Autodesk Inventor part; units mm, degrees
ref_plane "YZ Plane" through (0, 0, 0) normal (1, 0, 0) x (0, 1, 0)
ref_plane "XZ Plane" through (0, 0, 0) normal (0, 1, 0) x (-1, 0, 0)
ref_plane "XY Plane" through (0, 0, 0) normal (0, 0, 1) x (1, 0, 0)
sketch "Sketch1" plane through (0, 0, 0) normal (0, 0, 1) x (1, 0, 0)
  line L0 (-23.7998, 0) -> (0, 0)
  line L1 (0, 0) -> (0, -127)
  line L2 (0, -127) -> (-23.7998, -127)
  line L3 (-23.7998, -127) -> (-23.7998, 0)
  circle A0 centre (-11.0998, -12.7) radius 1.7859
  circle A1 centre (-11.0998, -38.1) radius 1.7859
  circle A2 centre (-11.0998, -63.5) radius 1.7859
  circle A3 centre (-11.0998, -88.9) radius 1.7859
  circle A4 centre (-11.0998, -114.3) radius 1.7859
  line L4 (-11.0998, -12.7) -> (-11.0998, -38.1) construction
  line L5 (-11.0998, -38.1) -> (-11.0998, -63.5) construction
  line L6 (-11.0998, -63.5) -> (-11.0998, -88.9) construction
  line L7 (-11.0998, -88.9) -> (-11.0998, -114.3) construction
  dimension "d0" = 23.7998
  dimension "d1" = 127
  dimension "d2" = 3.5719
  dimension "d3" = 25.4
  dimension "d4" = 12.7
  dimension "d5" = 11.0998
extrude "Extrusion1" add sketch "Sketch1" along normal blind 1.5875
sketch "Sketch3" plane through (0, -127, 0) normal (1, 0, 0) x (0, 0, -1)
  line L0 (-25.3873, 127) -> (-1.5875, 127)
  line L1 (-1.5875, 127) -> (-1.5875, 0)
  line L2 (-1.5875, 0) -> (-25.3873, 0)
  line L3 (-25.3873, 0) -> (-25.3873, 127)
  circle A0 centre (-12.6873, 114.3) radius 1.7859
  circle A1 centre (-12.6873, 88.9) radius 1.7859
  circle A2 centre (-12.6873, 63.5) radius 1.7859
  circle A3 centre (-12.6873, 38.1) radius 1.7859
  circle A4 centre (-12.6873, 12.7) radius 1.7859
  line L4 (-12.6873, 114.3) -> (-12.6873, 88.9) construction
  line L5 (-12.6873, 88.9) -> (-12.6873, 63.5) construction
  line L6 (-12.6873, 63.5) -> (-12.6873, 38.1) construction
  line L7 (-12.6873, 38.1) -> (-12.6873, 12.7) construction
  dimension "d8" = 23.7998
  dimension "d9" = 127
  dimension "d10" = 3.5719
  dimension "d11" = 25.4
  dimension "d12" = 12.7
  dimension "d13" = 11.0998
extrude "Extrusion2" add sketch "Sketch3" along normal blind 1.5875
sketch "Sketch4" plane through (0, -127, 1.5875) normal (0, -1, 0) x (1, 0, 0)
  line L0 (0, 0) -> (1.5875, 0)
  line L1 (0, 23.7998) -> (1.5875, 23.7998)
  line L2 (1.5875, 0) -> (0, -1.5875)
  line L3 (0, -1.5875) -> (0, 0)
extrude "Extrusion3" add sketch "Sketch4" against normal blind 127
properties part number "Angle bracket"
Could you check a few things on this model? Use its own coordinates, in mm. A direction names the side the tool comes from. Coordinates: 2 decimals unless noted, no trailing zeros. Loops run counter-clockwise (first coordinate to the right, second up) from the corner with the lowest first, then second, coordinate; pieces in that order, holes last. Notation, with made-up numbers: M 53.5,-7 L 65.5,-7 A18 cw 65.5,13 Z; hole C 56.5,-22.5 d3. An arc over 180 degrees is marked long. Put each result on its own line as item: value. Start each with the question number.
(1) Suppose I cut it at C-C on z = 18.5. Please give me the cut outline in (x, y), then the cut area to 3 significant figures.
(2) Thinking about a two-plate mould opening in Y: for faces 1 (the face through (0.78, -116.07, 12.92)), 2 (the face through (1.588, -63, 16)), 3 (the face through (-6, -127, 1)), which applies, pulls with the +Y half, pulls with the -Y half, needs draft (parallel to the pull), parting line crosses it, or undercut?
(3) Suppose I cut it at A-A on y = -88.9. Please give me the cut outline in (x, z), then the cut area to 3 significant figures.
(4) For faces 4 (the face through (-15, -63, 1.588)), 5 (the face through (0.78, -65.01, 11.73)), which set-ups out of +Z, -Z, +X, -X, +Y, -Y let a thin tool reach every point of the face, with its end or its side?
(5) I need wall thicknesses on line 1 (Z direction, x = -10.25, y = -31); line 2 (X direction, y = -88.9, z = 1.25). Which ranges of each line are inside material? Lowest first, please. Write a range as from..to.
(6) Will these pins go through, and if not, where does the flat tip stop? P1, Ø12, axis at x = -6, y = -104.5, coming from the -Z side; P2, Ø5.5, axis at y = -12.7, z = 12.69, coming from the -X side; P3, Ø3, axis at x = -11.1, y = -38.1, coming from the +Z side; P4, Ø1.5, axis at x = -7, y = -84, coming from the +Z side.
(7) Suppose I cut it at B-B on x = -11.5. Please give me the cut outline in (y, z), then the cut area to 3 significant figures.
(8) Suppose I cut it at D-D on y = -102.5. Please give me the cut outline in (x, z), then the cut area to 3 significant figures.
Solutions:
1. outline: M 0,-127 L 1.59,-127 L 1.59,0 L 0,0 Z
1. area: 202 mm2
2. face 1: undercut
2. face 2: needs draft
2. face 3: pulls with the -Y half
3. outline: M -23.8,0 L -12.89,0 L -12.89,1.59 L -23.8,1.59 Z; M -9.31,0 L 0,0 L 1.59,1.59 L 1.59,10.9 L 0,10.9 L 0,1.59 L -9.31,1.59 Z; M 0,14.47 L 1.59,14.47 L 1.59,25.39 L 0,25.39 Z
3. area: 65.5 mm2
4. face 4: +Z, -X, +Y, -Y
4. face 5: +X, -X
5. line 1: z = 0..1.59
5. line 2: x = -23.8..-12.89, -9.31..1.25
6. P1: stops at z = 0
6. P2: stops at x = 0
6. P3: passes through
6. P4: stops at z = 1.59
7. outline: M -127,0 L -116.04,0 L -116.04,1.59 L -127,1.59 Z; M -112.56,0 L -90.64,0 L -90.64,1.59 L -112.56,1.59 Z; M -87.16,0 L -65.24,0 L -65.24,1.59 L -87.16,1.59 Z; M -61.76,0 L -39.84,0 L -39.84,1.59 L -61.76,1.59 Z; M -36.36,0 L -14.44,0 L -14.44,1.59 L -36.36,1.59 Z; M -10.96,0 L 0,0 L 0,1.59 L -10.96,1.59 Z
7. area: 174 mm2
8. outline: M -23.8,0 L 0,0 L 1.59,1.59 L 1.59,25.39 L 0,25.39 L 0,1.59 L -23.8,1.59 Z
8. area: 76.8 mm2
